Source: CAD feature listing. Evaluate the final solid. Frame: model axes, mm. Face numbers are marked on the shaded views. A direction names the side the tool comes from. Coordinates: 2 decimals unless noted, no trailing zeros. Order: outer loops, then holes, each group sorted by start corner. A loop starts at its lowest first (then second) coordinate and runs counter-clockwise, first axis right, second up.
```python
from build123d import *

# Parameters (mm, degrees)
MAIN_DEPTH             = 25
SKETCH2_W              = 10
SKETCH2_H              = 10
VERTICALFORM_DEPTH     = 11
SKETCH3_R              = 1.5
MAKERBEAMFIXHOLE_DEPTH = 17
FILLET1_R              = 1


with BuildPart() as part:
    # Sketch1 → Main (new body)
    with BuildSketch(Plane.XY):
        Polygon((0, 10), (0, 6.45), (-1, 6.45), (-1, 3.55), (0, 3.55), (0, 0), (15, 0), (15, 10), align=None)
    extrude(amount=MAIN_DEPTH)

    # Sketch2 → VerticalForm (cut, through all)
    with BuildSketch(Plane(origin=(0, 0, 0), x_dir=(-1, 0, 0), z_dir=(0, -1, 0))):
        Polygon((1, -15), (1, -25), (-10, -25), (-10, -21.45), (-9, -21.45), (-9, -18.55), (-10, -18.55), (-10, -15), (-6.45, -15), (-6.45, -16), (-3.55, -16), (-3.55, -15), align=None)
        with Locations((-10, -5)):
            Rectangle(SKETCH2_W, SKETCH2_H)
    extrude(amount=-VERTICALFORM_DEPTH, mode=Mode.SUBTRACT)

    # Sketch3 → MakerBeamFixHole (cut, through all)
    with BuildSketch(Plane(origin=(15, 0, 0), x_dir=(0, 0, -1), z_dir=(1, 0, 0))):
        with Locations((-5, 5)):
            Circle(SKETCH3_R)
        with Locations((-20, 5)):
            Circle(SKETCH3_R)
    extrude(amount=-MAKERBEAMFIXHOLE_DEPTH, mode=Mode.SUBTRACT)

    # Fillet1
    fillet1_edges = [part.edges().sort_by_distance(p)[0] for p in [
        (5, 5, 10),
    ]]
    fillet(fillet1_edges, radius=FILLET1_R)


solid = part.part
```
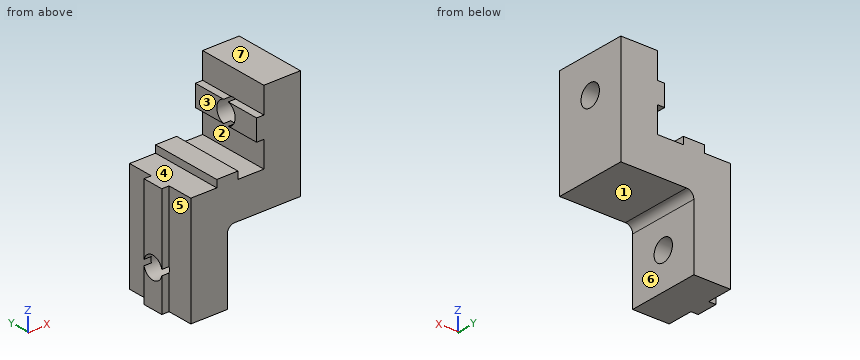
1. Draft query along X for the marked faces 1, 2 and 3. Return one class per face: released by +X, released by -X, zero draft, split by the parting line, or undercut.
Findings:
face 1: zero draft
face 2: undercut
face 3: released by -X
2. Ray query, line 1 (Z direction, x = 13.3, y = 5); line 2 (Y direction, x = 12.95, z = 20); line 3 (Z direction, x = 9.5, y = 9). Return the intervals inside material, ascending.
Findings:
line 1: z = 10 to 18.5, 21.5 to 25
line 2: y = 0 to 3.5, 6.5 to 10
line 3: z = 10 to 15, 18.55 to 21.45
3. Section query B-B on y = 5. Return loops of the section in (x, z).
Findings:
outline: (-1, 0) - (5, 0) - (5, 3.5) - (-1, 3.5) - close; (-1, 6.5) - (5, 6.5) - (5, 9) arc R1 cw to (6, 10) - (15, 10) - (15, 18.5) - (10, 18.5) - (10, 15) - (6.45, 15) - (6.45, 16) - (3.55, 16) - (3.55, 15) - (-1, 15) - close; (10, 21.5) - (15, 21.5) - (15, 25) - (10, 25) - close
4. Section query C-C on x = 2.5. Return loops of the section in (y, z), plus the area to 3 significant figures.
Findings:
outline: (0, 0) - (10, 0) - (10, 15) - (0, 15) - close; hole circle Ø3 at (5, 5)
area: 143 mm2
5. Access query for the marked faces 4, 5, 6 and 7. Directions: +Z, -Z, +X, -X, +Y, -Y. A direction counts if a zero-diameter tool reaches every point of the face in a straight line with its end or side. Return the directions, or none.
Findings:
face 4: +Z, -X, +Y, -Y
face 5: +Z, -Z, -X, -Y
face 6: -Z, +X, +Y, -Y
face 7: +Z, +X, -X, +Y, -Y
6. Section query D-D on y = 7.75. Return loops of the section in (x, z).
Findings:
outline: (0, 0) - (5, 0) - (5, 9) arc R1 cw to (6, 10) - (15, 10) - (15, 25) - (10, 25) - (10, 21.45) - (9, 21.45) - (9, 18.55) - (10, 18.55) - (10, 15) - (6.45, 15) - (6.45, 16) - (3.55, 16) - (3.55, 15) - (0, 15) - close
7. Pin query (flat end, axial travel): P1, Ø2.5, axis at y = 6.5, z = 2.5, coming from the +X side; P2, Ø2.5, axis at x = 0.5, y = 4, coming from the +Z side; P3, Ø1.8, axis at y = 4.5, z = 23, coming from the -X side; P4, Ø1.1, axis at x = -0.5, z = 11, coming from the +Y side. Return the tip coordinate at first contact, or that it passes through.
Findings:
P1: stops at x = 5
P2: stops at z = 15
P3: stops at x = 10
P4: stops at y = 10
8. Section query A-A on z = 5. Return loops of the section in (x, y).
Findings:
outline: (0, 0) - (5, 0) - (5, 3.5) - (0, 3.5) - close; (0, 6.5) - (5, 6.5) - (5, 10) - (0, 10) - close
